Source: CAD feature listing. Evaluate the final solid. Frame: model axes, mm. Face numbers are marked on the shaded views. A direction names the side the tool comes from. Coordinates: 2 decimals unless noted, no trailing zeros. Write each loop counter-clockwise with the first axis right and the second up, starting at its lowest first coordinate (ties: lowest second). Pieces come first, ordered by that corner, then holes. Notation, with made-up numbers: (86.5, 29) - (97.5, 29) arc R15 ccw to (97.5, 39) - close; hole circle Ø5 at (6, 57). An arc over 180 degrees is marked (long way). One line per item, written item: value.
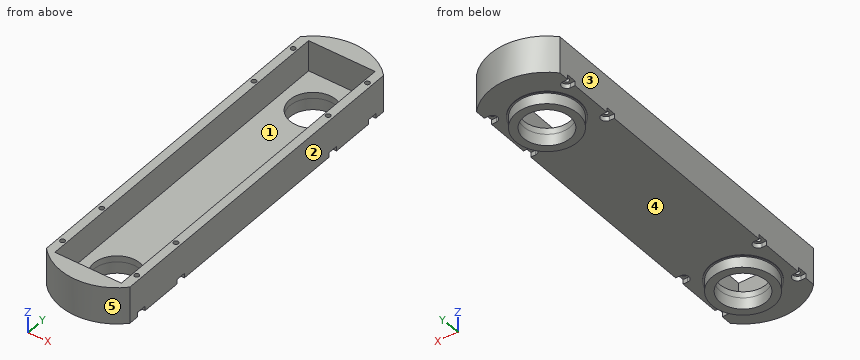
from build123d import *

# Parameters (mm, degrees)
SKETCH_1_W          = 54
SKETCH_1_H          = 220
EXTRUDE_1_DEPTH     = 24
SKETCH_2_R          = 1.55
CUT_EXTRUDE_1_DEPTH = 25
EXTRUDE_2_DEPTH     = 24
SKETCH_5_W          = 43
SKETCH_5_H          = 220
CUT_EXTRUDE_3_DEPTH = 20
CUT_EXTRUDE_4_DEPTH = 3
SKETCH_7_R          = 15
CUT_EXTRUDE_5_DEPTH = 25
SKETCH_11_R         = 20
SKETCH_11_R_2       = 15
EXTRUDE_3_DEPTH     = 7.5
SKETCH_12_R         = 21
SKETCH_12_R_2       = 20
EXTRUDE_4_DEPTH     = 0.5


with BuildPart() as part:
    # 草图1 → 凸台-拉伸1 (new body)
    with BuildSketch(Plane.XY):
        Rectangle(SKETCH_1_W, SKETCH_1_H)
    extrude(amount=EXTRUDE_1_DEPTH)

    # 草图2 → 切除-拉伸1 (cut, through all)
    with BuildSketch(Plane.XY.offset(24)):
        with Locations((-24, 100)):
            Circle(SKETCH_2_R)
        with Locations((24, 100)):
            Circle(SKETCH_2_R)
        with Locations((24, 66)):
            Circle(SKETCH_2_R)
        with Locations((-24, 66)):
            Circle(SKETCH_2_R)
        with Locations((24, -100)):
            Circle(SKETCH_2_R)
        with Locations((24, -66)):
            Circle(SKETCH_2_R)
        with Locations((-24, -66)):
            Circle(SKETCH_2_R)
        with Locations((-24, -100)):
            Circle(SKETCH_2_R)
    extrude(amount=-CUT_EXTRUDE_1_DEPTH, mode=Mode.SUBTRACT)

    # 草图3 → 凸台-拉伸2 (add)
    with BuildSketch(Plane.XY.offset(24)):
        with BuildLine():
            Line((-27, 110), (27, 110))
            ThreePointArc((27, 110), (0, 121.795200461), (-27, 110))
        make_face()
        with BuildLine():
            Line((-27, -110), (27, -110))
            ThreePointArc((27, -110), (0, -121.795200461), (-27, -110))
        make_face()
    extrude(amount=-EXTRUDE_2_DEPTH)

    # 草图5 → 切除-拉伸3 (cut)
    with BuildSketch(Plane.XY.offset(24)):
        Rectangle(SKETCH_5_W, SKETCH_5_H)
    extrude(amount=-CUT_EXTRUDE_3_DEPTH, mode=Mode.SUBTRACT)

    # 草图6 → 切除-拉伸4 (cut)
    with BuildSketch(Plane(origin=(0, 0, 0), x_dir=(-1, 0, 0), z_dir=(0, 0, -1))):
        with BuildLine():
            Line((-27, 69.2), (-24, 69.2))
            ThreePointArc((-24, 69.2), (-20.8, 66), (-24, 62.8))
            Line((-24, 62.8), (-27, 62.8))
            Line((-27, 62.8), (-27, 69.2))
        make_face()
        with BuildLine():
            Line((-27, 103.2), (-27, 96.8))
            Line((-27, 96.8), (-24, 96.8))
            ThreePointArc((-24, 96.8), (-20.8, 100), (-24, 103.2))
            Line((-24, 103.2), (-27, 103.2))
        make_face()
        with BuildLine():
            Line((27, 69.2), (24, 69.2))
            ThreePointArc((24, 69.2), (20.8, 66), (24, 62.8))
            Line((24, 62.8), (27, 62.8))
            Line((27, 62.8), (27, 69.2))
        make_face()
        with BuildLine():
            Line((27, 103.2), (24, 103.2))
            ThreePointArc((24, 103.2), (20.8, 100), (24, 96.8))
            Line((24, 96.8), (27, 96.8))
            Line((27, 96.8), (27, 103.2))
        make_face()
        with BuildLine():
            Line((27, -69.2), (27, -62.8))
            Line((27, -62.8), (24, -62.8))
            ThreePointArc((24, -62.8), (20.8, -66), (24, -69.2))
            Line((24, -69.2), (27, -69.2))
        make_face()
        with BuildLine():
            Line((27, -103.2), (27, -96.8))
            Line((27, -96.8), (24, -96.8))
            ThreePointArc((24, -96.8), (20.8, -100), (24, -103.2))
            Line((24, -103.2), (27, -103.2))
        make_face()
        with BuildLine():
            Line((-27, -103.2), (-24, -103.2))
            ThreePointArc((-24, -103.2), (-20.8, -100), (-24, -96.8))
            Line((-24, -96.8), (-27, -96.8))
            Line((-27, -96.8), (-27, -103.2))
        make_face()
        with BuildLine():
            Line((-27, -69.2), (-24, -69.2))
            ThreePointArc((-24, -69.2), (-20.8, -66), (-24, -62.8))
            Line((-24, -62.8), (-27, -62.8))
            Line((-27, -62.8), (-27, -69.2))
        make_face()
    extrude(amount=-CUT_EXTRUDE_4_DEPTH, mode=Mode.SUBTRACT)

    # 草图7 → 切除-拉伸5 (cut, through all)
    with BuildSketch(Plane(origin=(0, 0, 0), x_dir=(-1, 0, 0), z_dir=(0, 0, -1))):
        with Locations((0, 85)):
            Circle(SKETCH_7_R)
        with Locations((0, -85)):
            Circle(SKETCH_7_R)
    extrude(amount=-CUT_EXTRUDE_5_DEPTH, mode=Mode.SUBTRACT)

    # 草图11 → 凸台-拉伸3 (add)
    with BuildSketch(Plane(origin=(0, 0, 0), x_dir=(-1, 0, 0), z_dir=(0, 0, -1))):
        with Locations((0, 85)):
            Circle(SKETCH_11_R)
        with Locations((0, 85)):
            Circle(SKETCH_11_R_2, mode=Mode.SUBTRACT)
        with Locations((0, -85)):
            Circle(SKETCH_11_R)
        with Locations((0, -85)):
            Circle(SKETCH_11_R_2, mode=Mode.SUBTRACT)
    extrude(amount=EXTRUDE_3_DEPTH)

    # 草图12 → 凸台-拉伸4 (add)
    with BuildSketch(Plane(origin=(0, 0, 0), x_dir=(-1, 0, 0), z_dir=(0, 0, -1))):
        with Locations((0, 85)):
            Circle(SKETCH_12_R)
        with Locations((0, 85)):
            Circle(SKETCH_12_R_2, mode=Mode.SUBTRACT)
        with Locations((0, -85)):
            Circle(SKETCH_12_R)
        with Locations((0, -85)):
            Circle(SKETCH_12_R_2, mode=Mode.SUBTRACT)
    extrude(amount=EXTRUDE_4_DEPTH)


solid = part.part
1) Section query A-A on x = 0. State how many separate pieces and enclosed holes the cut face has, then the cut area to 3 significant figures.
Values found:
separate pieces: 3
enclosed holes: 0
area: 1,360 mm2
2) Draft query along Y for the marked faces 3, 4 and 5. Return one class per face: released by +Y, released by -Y, zero draft, split by the parting line, or undercut.
Values found:
face 3: zero draft
face 4: undercut
face 5: released by -Y
3) Reachability of the marked faces 1 and 2 from +Z, -Z, +X, -X, +Y, -Y: full face, straight path, thin tool, end or side. Return the list, or none.
Values found:
face 1: +Z
face 2: +Z, -Z, +X, +Y, -Y
4) Contact query for flat-ended pins moving along their axis: P1, Ø12, axis at x = -10, z = 16, coming from the -Y side; P2, Ø3, axis at x = 24.5, y = -65, coming from the -Z side; P3, Ø8, axis at x = 1.5, z = 4, coming from the -Y side. Output: stop coordinate, or through.
Values found:
P1: y = -121.58
P2: z = 3
P3: y = -121.8
5) Section query B-B on y = -85. Output: boundary loops of the cut face in (x, z).
Values found:
outline: (-27, 0) - (-21, 0) - (-21, -0.5) - (-20, -0.5) - (-20, -7.5) - (-15, -7.5) - (-15, 4) - (-21.5, 4) - (-21.5, 24) - (-27, 24) - close; (15, -7.5) - (20, -7.5) - (20, -0.5) - (21, -0.5) - (21, 0) - (27, 0) - (27, 24) - (21.5, 24) - (21.5, 4) - (15, 4) - close
6) Material intervals for line 1 (X direction, y = 66, z = 18.75); line 2 (Y direction, x = 0, z = -4); line 3 (Y direction, x = -25, z = 7), sorted ascending.
Values found:
line 1: -27 to -25.55, -22.45 to -21.5, 21.5 to 22.45, 25.55 to 27
line 2: -105 to -100, -70 to -65, 65 to 70, 100 to 105
line 3: -112 to -101.18, -98.82 to -67.18, -64.82 to 64.82, 67.18 to 98.82, 101.18 to 112
7) Section query D-D on y = 60. Output: boundary loops of the cut face in (x, z).
Values found:
outline: (-27, 0) - (27, 0) - (27, 24) - (21.5, 24) - (21.5, 4) - (-21.5, 4) - (-21.5, 24) - (-27, 24) - close
